from build123d import *

# Parameters (mm, degrees)
F1_DEPTH = 76.2
F2_R     = 76.2
F3_R     = 76.19999
F5_R     = 12.7
F6_DEPTH = 152.4
F4_R     = 22.225
F7_DEPTH = 76.2


# Not quite as in the source:
# - a fillet or chamfer is up to 0.001 mm smaller than in the source, because OpenCascade refuses the exact size


with BuildPart() as f1:
    # F0 (on Top) → F1 (new body)
    with BuildSketch(Plane.XY):
        Polygon((0, 152.4), (0, 0), (225.425, 0), (225.425, 50.8), (149.225, 50.8), (149.225, 101.6), (225.425, 101.6), (225.425, 152.4), align=None)
    extrude(amount=F1_DEPTH)

    # F2
    f2_edges = [f1.edges().sort_by_distance(p)[0] for p in [
        (0, 152.4, 38.1),
    ]]
    fillet(f2_edges, radius=F2_R)

    # F3 (radius 76.2 in the source; OpenCascade refuses exactly that, so slightly less here)
    f3_edges = [f1.edges().sort_by_distance(p)[0] for p in [
        (0, 0, 38.1),
    ]]
    fillet(f3_edges, radius=F3_R)

    # F5 (on face) → F6 (cut)
    with BuildSketch(Plane(origin=(0, 152.4, 0), x_dir=(-1, 0, 0), z_dir=(0, 1, 0))):
        with Locations((-187.325, 38.1)):
            Circle(F5_R)
    extrude(amount=-F6_DEPTH, mode=Mode.SUBTRACT)

    # F4 (on face) → F7 (cut)
    with BuildSketch(Plane.XY.offset(76.2)):
        with Locations((111.125, 76.2)):
            Circle(F4_R)
    extrude(amount=-F7_DEPTH, mode=Mode.SUBTRACT)


solid = f1.part
CAD build for the part. Positions are in the model's coordinates, mm. A direction names the side the tool comes from. Give positions to 0.01 mm unless a question says otherwise; leave off trailing zeros. Order: outer loops, then holes, each group sorted by start corner. A loop starts at its lowest first (then second) coordinate and runs counter-clockwise, first axis right, second up. Notation, with made-up numbers: (72.25, -4.75) - (119.25, -4.75) arc R28 ccw to (119.25, 24.25) - close; hole circle Ø9 at (-6, 66). An arc over 180 degrees is marked (long way). Write each question's results on one line, items separated by ' | '.
1. Saw through at D-D on x = 110. List the corners of the cut face in (y, z).
Calculated:
outline: (0, 0) - (54, 0) - (54, 76.2) - (0, 76.2) - close; (98.4, 0) - (152.4, 0) - (152.4, 76.2) - (98.4, 76.2) - close
2. Pull direction Y, two halves, no side cores. Call faces 3 (the face through (225.425, 25, 38)), 4 (the face through (150, 0, 38)), 5 (the face through (131.655, 67.688, 38.633)): released by +Y, released by -Y, zero draft, split by the parting line, or undercut.
Calculated:
face 3: zero draft | face 4: released by -Y | face 5: undercut
3. Saw through at B-B on y = 82.5. List the corners of the cut face in (x, z) (3 decimals), and give its area (3 significant figures).
Calculated:
outline: (0.261, 0) - (89.812, 0) - (89.812, 76.2) - (0.261, 76.2) - close; (132.438, 0) - (149.225, 0) - (149.225, 76.2) - (132.438, 76.2) - close | area: 8,100 mm2
4. Saw through at A-A on z = 38.1. Count the separate pieces of the cut face and the enclosed holes in it, and give its area (3 significant figures).
Calculated:
separate pieces: 3 | enclosed holes: 1 | area: 23,900 mm2
5. 3-axis set-ups, long thin cutter, end or side, ignore diameter. For faces 1 (the face through (225.425, 127, 38)), 2 (the face through (205, 50.8, 38)): which of +Z, -Z, +X, -X, +Y, -Y reach the whole face in a straight line?
Calculated:
face 1: +Z, -Z, +X, +Y, -Y | face 2: +Z, -Z, +X
6. Probe L1, parallel to Y at x = 111, z = 23; L2, parallel to Y at x = 203, z = 69; L3, parallel to Z at x = 183, y = 144. List the from-to ranges inside material, lowest first. Write a range as from..to.
Calculated:
L1: y = 0..53.98, 98.42..152.4 | L2: y = 0..50.8, 101.6..152.4 | L3: z = 0..26.16, 50.04..76.2
7. Pin check, flat tips, straight feed: pin 1 (6 mm diameter, centred on x = 184, y = 127, fed in from -Z); pin 2 (12 mm diameter, centred on y = 63, z = 47, fed in from -X); pin 3 (5 mm diameter, centred on x = 45, z = 29.5, fed in from +Y); pin 4 (15 mm diameter, centred on y = 87, z = 37, fed in from +X) (3 decimals). Stop position of each tip, or through.
Calculated:
pin 1: stops at z = 0 | pin 2: stops at x = 0.34 | pin 3: stops at y = 146.79 | pin 4: stops at x = 149.225
